Verification items for the finished model (mm, model axes). Face numbers are marked on the shaded views. A direction names the side the tool comes from. Coordinates: 2 decimals unless noted, no trailing zeros. Loops run counter-clockwise (first coordinate to the right, second up) from the corner with the lowest first, then second, coordinate; pieces in that order, holes last. Notation, with made-up numbers: (24, -24) -> (33, -24) arc R9 cw to (33, -9) -> close; hole circle Ø8 at (19, -14). An arc over 180 degrees is marked (long way). Answer as a JSON object with one key per item and string values. Group by question number.
Q1. Cross-section at C-C on y = 28. Give the number of separate pieces and of enclosed holes in the cut face, and give its area (3 significant figures).
Q2. Cross-section at A-A on x = 250. Record the boundary of the cut face in (y, z).
Q3. Scan lines: L1, parallel to Z at x = 0, y = 19.5; L2, parallel to Z at x = 0.5, y = 26; L3, parallel to Y at x = 66, z = 19.5. Record each from-to range of solid material in increasing order.
Q4. Release check for a two-part mould opening along Y. For the marked faces 3, 4 and 5 record: released by +Y, released by -Y, zero draft, split by the parting line, or undercut.
Q5. Set-up check for the marked faces 1 and 2: record each of +Z, -Z, +X, -X, +Y, -Y from which the full face is reachable in a straight line by a thin tool's end or side.
Q6. Cross-section at B-B on x = 47. Record the boundary of the cut face in (y, z).
Q7. Gauge pin test, flat ends, axial feed: pin 1 Ø8 at (x, y) = (69, 28) entering from +Z; pin 2 Ø8 at (x, y) = (20.5, 21.5) entering from +Z; pin 3 Ø12 at (x, z) = (57.5, -23) entering from +Y; pin 4 Ø3 at (x, z) = (130, 7.31) entering from +Y. Record the tip position at first contact, or that the pin passes through.
Q8. Cross-section at D-D on x = -19.5. Record the boundary of the cut face in (y, z).
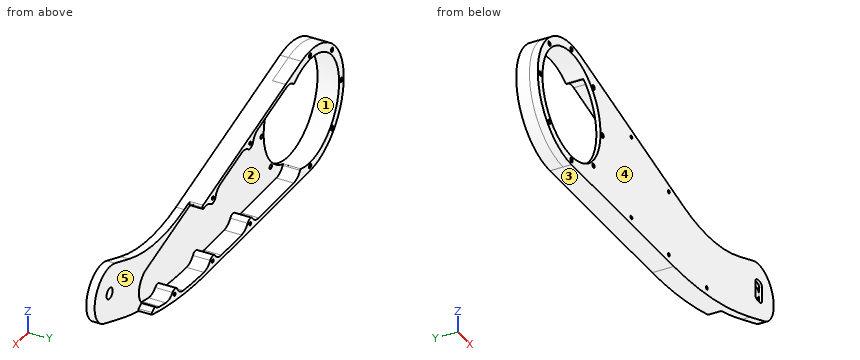
```python
from build123d import *

# Parameters (mm, degrees)
EXTRUDE_1_DEPTH             = 9.500000000000002
EXTRUDE_2_DEPTH             = 115.05569061587602
EXTRUDE_3_DEPTH             = 5.999999999999999
CUT_EXTRUDE_1_DEPTH         = 3.000000000000001
EXTRUDE_4_DEPTH             = 12.5
EXTRUDE_5_DEPTH             = 12.5
EXTRUDE_START               = 12.5
EXTRUDE_6_DEPTH             = 12.5
EXTRUDE_7_DEPTH             = 12.5
CUT_EXTRUDE_2_DEPTH         = 2
HOLE_WIZARD_8_0_8_1_D       = 8
HOLE_WIZARD_8_0_8_1_DEPTH   = 6
HOLE_WIZARD_2_5_2_5_1_D     = 2.5
HOLE_WIZARD_3_2_3_2_1_D     = 3.2
HOLE_WIZARD_3_2_3_2_1_DEPTH = 15.5
HOLE_WIZARD_3_2_3_2_2_D     = 3.2
FILLET_1_R                  = 1
FILLET_2_R                  = 2
FILLET_3_R                  = 120.00000000000003


with BuildPart() as part:
    # Эскиз1 → Бобышка-Вытянуть1 (new body)
    with BuildSketch(Plane.XZ):
        with BuildLine():
            Line((31.779364408196322, 35.09465055833703), (32.53928446481828, 37.996808635931096))
            Line((32.53928446481828, 37.996808635931096), (11.398800849455474, 43.53237116439277))
            ThreePointArc((11.398800849455474, 43.53237116439277), (-44.6315846816897, 5.746446623885336), (0, -45))
            Line((0, -45), (136.6047385645944, -45))
            ThreePointArc((136.6047385645944, -45), (174.0514558866368, -42.49971682694584), (210.833370462018, -35.04325558103525))
            ThreePointArc((210.833370462018, -35.04325558103525), (211.56166337980483, -34.20622038377409), (211.068983168903, -33.2120852293116))
            Line((211.068983168903, -33.2120852293116), (207.14834257891937, -30.95366812818016))
            ThreePointArc((207.14834257891937, -30.95366812818016), (204.26320644859996, -33.162341546064276), (200.87949883001698, -34.4862643192222))
            ThreePointArc((200.87949883001698, -34.4862643192222), (171.45991408687433, -39.811616665453215), (141.6391276395998, -41.95452117487615))
            ThreePointArc((141.6391276395998, -41.95452117487615), (136.9266537788762, -40.870335373727656), (133.2738484900434, -37.7017580492345))
            ThreePointArc((133.2738484900434, -37.7017580492345), (129.99235706441334, -36.0000073018108), (126.71739277340599, -37.7142857142829))
            ThreePointArc((126.71739277340599, -37.7142857142829), (123.13997520578543, -40.86405260427835), (118.5108747069212, -42))
            Line((118.5108747069212, -42), (21.853203426500148, -42))
            ThreePointArc((21.853203426500148, -42), (16.621968089397427, -40.52256867662841), (12.936490941687484, -36.52683536956956))
            ThreePointArc((12.936490941687484, -36.52683536956956), (38.432753475903155, -4.948329037205795), (21.767072161661147, 32.05865046300353))
            ThreePointArc((21.767072161661147, 32.05865046300353), (26.34449721336863, 34.99051102645374), (31.779364408196322, 35.09465055833703))
        make_face()
    extrude(amount=-EXTRUDE_1_DEPTH)

    # Эскиз2 → Бобышка-Вытянуть2 (add)
    with BuildSketch(Plane(origin=(21.140483615362722, 0, -5.535562528461676), x_dir=(-0.2533066855420127, 0, -0.967386025875772), z_dir=(0.9673860258757722, 0, -0.2533066855420127))):
        Polygon((-42.00000000000173, 0), (-45.000000000001705, -8.7e-16), (-45.000000000001705, 9.5), (-42.00000000000173, 9.5), align=None)
    extrude(amount=EXTRUDE_2_DEPTH)

    # Эскиз3 → Бобышка-Вытянуть3 (add)
    with BuildSketch(Plane(origin=(0, 9.500000000000002, 0), x_dir=(-1, 0, 0), z_dir=(0, 1, 0))):
        with BuildLine():
            Line((0, -45), (-136.6047385645944, -45))
            ThreePointArc((-136.6047385645944, -45), (-188.48995572376379, -40.179977983128), (-238.599420052963, -25.88487544631455))
            Line((-238.599420052963, -25.88487544631455), (-257.242147749639, -18.6427276966758))
            ThreePointArc((-257.242147749639, -18.6427276966758), (-268.6427276966758, 7.242147749639007), (-242.757852250361, 18.6427276966758))
            Line((-242.757852250361, 18.6427276966758), (-187.87549846851005, -2.677441830178293))
            Line((-187.87549846851005, -2.677441830178293), (-11.398800849390101, 43.53237116440985))
            ThreePointArc((-11.398800849390101, 43.53237116440985), (44.63158468169398, 5.74644662385182), (0, -45))
        make_face()
    extrude(amount=EXTRUDE_3_DEPTH)

    # Эскиз4 → Вырез-Вытянуть1 (cut)
    with BuildSketch(Plane.XZ.offset(-9.500000000000002)):
        with BuildLine():
            Line((201.174054751897, -9.26076332158908), (31.779364408181, 35.094650558340646))
            ThreePointArc((31.779364408181, 35.094650558340646), (26.344497213361088, 34.99051102645149), (21.767072161661147, 32.05865046300353))
            ThreePointArc((21.767072161661147, 32.05865046300353), (38.432753475903155, -4.9483290372057915), (12.936490941687483, -36.526835369569554))
            ThreePointArc((12.936490941687483, -36.526835369569554), (16.621968089397427, -40.52256867662841), (21.853203426500148, -42))
            Line((21.853203426500148, -42), (118.5108747069212, -42))
            ThreePointArc((118.5108747069212, -42), (123.13997520578546, -40.8640526042784), (126.71739277340599, -37.7142857142829))
            ThreePointArc((126.71739277340599, -37.7142857142829), (129.99235706441334, -36.00000730181071), (133.2738484900434, -37.7017580492345))
            ThreePointArc((133.2738484900434, -37.7017580492345), (136.92665377887585, -40.870335373728324), (141.6391276395998, -41.95452117487615))
            ThreePointArc((141.6391276395998, -41.95452117487615), (171.4599140868743, -39.8116166654531), (200.87949883001698, -34.4862643192222))
            ThreePointArc((200.87949883001698, -34.4862643192222), (210.88018165389494, -21.98857114883415), (201.174054751897, -9.26076332158908))
        make_face()
    extrude(amount=-CUT_EXTRUDE_1_DEPTH, mode=Mode.SUBTRACT)

    # Эскиз5 → Бобышка-Вытянуть4 (add)
    with BuildSketch(Plane.XZ.offset(-12.500000000000002)):
        with BuildLine():
            Line((69.39219411302629, 25.245861169673617), (91.62103262914168, 19.425316674141865))
            ThreePointArc((91.62103262914168, 19.425316674141865), (86.85516242440718, 19.49899914179931), (82.59656164963481, 17.358142454506996))
            ThreePointArc((82.59656164963481, 17.358142454506996), (78.98677325783201, 16.531272766653025), (76.24546493074466, 19.02115516751604))
            ThreePointArc((76.24546493074466, 19.02115516751604), (73.58257817824061, 22.974379428515537), (69.39219411302629, 25.245861169673617))
        make_face()
    extrude(amount=EXTRUDE_4_DEPTH)

    # Эскиз6 → Бобышка-Вытянуть5 (add)
    with BuildSketch(Plane.XZ.offset(-12.500000000000002)):
        with BuildLine():
            Line((119.39219411302322, 12.153534075498996), (141.6210326291386, 6.332989579967239))
            ThreePointArc((141.6210326291386, 6.332989579967239), (136.8551624244041, 6.406672047624693), (132.59656164963178, 4.26581536033236))
            ThreePointArc((132.59656164963178, 4.26581536033236), (128.986773257829, 3.438945672478428), (126.24546493074165, 5.928828073341451))
            ThreePointArc((126.24546493074165, 5.928828073341451), (123.58257817823758, 9.882052334340969), (119.39219411302322, 12.153534075498996))
        make_face()
    extrude(amount=EXTRUDE_5_DEPTH)

    # Эскиз7 → Бобышка-Вытянуть6 (add)
    with BuildSketch(Plane.XZ.offset(-12.500000000000002).offset(EXTRUDE_START)):
        with BuildLine():
            ThreePointArc((169.350540410565, -40.06937238400199), (173.90141926099287, -38.33703307937142), (177.09458850993005, -34.660734951460455))
            ThreePointArc((177.09458850993005, -34.660734951460455), (180.02526915777943, -32.52060975329769), (183.4802160115175, -33.63073008971875))
            ThreePointArc((183.4802160115175, -33.63073008971875), (187.66734322037206, -36.11658276325075), (192.5321018049815, -36.33017511120823))
            ThreePointArc((192.5321018049815, -36.33017511120823), (180.98072250488946, -38.44404700724877), (169.350540410565, -40.06937238400199))
        make_face()
    extrude(amount=-EXTRUDE_6_DEPTH)

    # Эскиз8 → Бобышка-Вытянуть7 (add)
    with BuildSketch(Plane.XZ.offset(-12.500000000000002)):
        with BuildLine():
            Line((91.489125293076, -42), (68.510874706924, -42))
            ThreePointArc((68.510874706924, -42), (73.13997520578674, -40.86405260427919), (76.71739277340684, -37.714285714285715))
            ThreePointArc((76.71739277340684, -37.714285714285715), (80.00000000000003, -36), (83.2826072265932, -37.714285714285765))
            ThreePointArc((83.2826072265932, -37.714285714285765), (86.86002479421332, -40.86405260427916), (91.489125293076, -42))
        make_face()
    extrude(amount=EXTRUDE_7_DEPTH)

    # Эскиз9 → Вырез-Вытянуть2 (cut)
    with BuildSketch(Plane(origin=(0, 15.5, 0), x_dir=(-1, 0, 0), z_dir=(0, 1, 0))):
        with BuildLine():
            Line((-245.75, -6.777720855862977), (-245.75, 6.777720855862977))
            ThreePointArc((-245.75, 6.777720855862977), (-249.99999999999997, 7.999999999999998), (-254.24999999999997, 6.777720855862994))
            Line((-254.24999999999997, 6.777720855862994), (-254.24999999999997, -6.777720855862994))
            ThreePointArc((-254.24999999999997, -6.777720855862994), (-249.99999999999997, -7.999999999999997), (-245.75, -6.777720855862977))
        make_face()
    extrude(amount=-CUT_EXTRUDE_2_DEPTH, mode=Mode.SUBTRACT)

    # Эскиз10 → Вырез-Повернуть1 (revolve, cut)
    with BuildSketch(Plane(origin=(0, 0, 0), x_dir=(-1, 0, 0), z_dir=(0, 0, -1)), mode=Mode.PRIVATE) as cut_revolve_1_sk:
        Polygon((-38.75000000000001, 0), (0, 0), (0, 15.5), (-38.75, 15.5), align=None)
    revolve(cut_revolve_1_sk.sketch.rotate(Axis((0, 0, 0), (0, 1, 0)), 270), axis=Axis((0, 0, 0), (0, 1, 0)), mode=Mode.SUBTRACT)

    # Диаметр отверстия Ø8.0 (8)1
    with Locations(Plane(origin=(0, 9.500000000000002, 0), x_dir=(-1, 0, 0), z_dir=(0, -1, 0))):
        with Locations((-250, 0)):
            Hole(HOLE_WIZARD_8_0_8_1_D / 2, depth=HOLE_WIZARD_8_0_8_1_DEPTH)

    # Диаметр отверстия Ø2.5 (2.5)1 (through all)
    with Locations(Plane(origin=(0, 15.5, 0), x_dir=(1, 0, 0), z_dir=(0, 1, 0))):
        with Locations((130, -7.308489776), (130, 40), (80, -20.40081687), (180.662238056, 36.469567923), (80, 40)):
            Hole(HOLE_WIZARD_2_5_2_5_1_D / 2)

    # Диаметр отверстия Ø3.2 (3.2)1
    with Locations(Plane(origin=(0, 15.5, 0), x_dir=(1, 0, 0), z_dir=(0, 1, 0))):
        with Locations((29.344931419, 29.344931419), (41.5, 0), (29.344931419, -29.344931419)):
            Hole(HOLE_WIZARD_3_2_3_2_1_D / 2, depth=HOLE_WIZARD_3_2_3_2_1_DEPTH)

    # Диаметр отверстия Ø3.2 (3.2)2 (through all)
    with Locations(Plane(origin=(0, 15.5, 0), x_dir=(1, 0, 0), z_dir=(0, 1, 0))):
        with Locations((-29.344931419, 29.344931419), (0, 41.5), (0, -41.5), (-29.344931419, -29.344931419), (-41.5, 0)):
            Hole(HOLE_WIZARD_3_2_3_2_2_D / 2)

    # Скругление1
    fillet_1_edges = [part.edges().sort_by_distance(p)[0] for p in [
        (21.767072161661147, 6.250000000000002, 32.05865046300353),
        (12.936490941687481, 6.250000000000002, -36.526835369569554),
        (207.14834257891937, 4.750000000000001, -30.953668128180162),
        (143.08263170741236, 4.75, 5.95027491566762),
        (143.84255176403838, 4.749999999999999, 8.852432993294912),
    ]]
    fillet(fillet_1_edges, radius=FILLET_1_R)

    # Скругление2
    fillet_2_edges = [part.edges().sort_by_distance(p)[0] for p in [
        (245.75, 14.5, -6.777720855862977),
        (254.24999999999997, 14.5, -6.777720855862994),
        (254.24999999999997, 14.5, 6.777720855862995),
        (245.75, 14.5, 6.7777208558629765),
    ]]
    fillet(fillet_2_edges, radius=FILLET_2_R)

    # Скругление3
    fillet_3_edges = [part.edges().sort_by_distance(p)[0] for p in [
        (187.87549846851005, 12.500000000000002, -2.677441830178293),
    ]]
    fillet(fillet_3_edges, radius=FILLET_3_R)


with BuildPart() as body_2:
    # Зеркальное отражение1: mirrored copy
    add(part.part.mirror(Plane(origin=(0, 15.5, 0), x_dir=(0, 0, 1), z_dir=(0, -1, 0))))


solid = body_2.part
```
Computed values:
{
 "1": {"separate pieces": "1", "enclosed holes": "10", "area": "2,290 mm²"},
 "2": {"outline": "(15.5, -21.46) -> (21.5, -21.46) -> (21.5, -4) -> (17.5, -4) -> (17.5, -8) -> (15.5, -8) -> close; (15.5, 8) -> (17.5, 8) -> (17.5, 4) -> (21.5, 4) -> (21.5, 20) -> (15.5, 20) -> close"},
 "3": {"L1": "z = -45 to -43.1, -39.9 to -38.75, 38.75 to 39.9, 43.1 to 45", "L2": "z = -45 to -43.02, -39.98 to -38.75, 38.75 to 39.98, 43.02 to 45", "L3": "y = 15.5 to 18.5"},
 "4": {"face 3": "zero draft", "face 4": "released by -Y", "face 5": "released by +Y"},
 "5": {"face 1": "+Y, -Y", "face 2": "+Y"},
 "6": {"outline": "(15.5, -45) -> (31, -45) -> (31, -42) -> (18.5, -42) -> (18.5, 31.11) -> (31, 31.11) -> (31, 34.21) -> (15.5, 34.21) -> close"},
 "7": {"pin 1": "stops at z = 29.5", "pin 2": "stops at z = 42.2", "pin 3": "stops at y = 18.5", "pin 4": "stops at y = 31"},
 "8": {"outline": "(15.5, -40.56) -> (31, -40.56) -> (31, -33.49) -> (15.5, -33.49) -> close; (15.5, 33.49) -> (31, 33.49) -> (31, 40.56) -> (15.5, 40.56) -> close"}
}
